Part print with two shaded views. Sizes in mm from the minimum x, y, z corner. A direction names the side the tool comes from. Round coordinates to 2 decimals unless told otherwise and drop trailing zeros. Write each loop counter-clockwise with the first axis right and the second up, starting at its lowest first coordinate (ties: lowest second). Pieces come first, ordered by that corner, then holes. Notation, with made-up numbers: (-32, 1) -> (-15, 1) arc R31 ccw to (-15, 37) -> close; hole circle Ø2 at (-33.5, -35.5). An arc over 180 degrees is marked (long way). Answer in a Markdown table with one row per item. Add a question column.
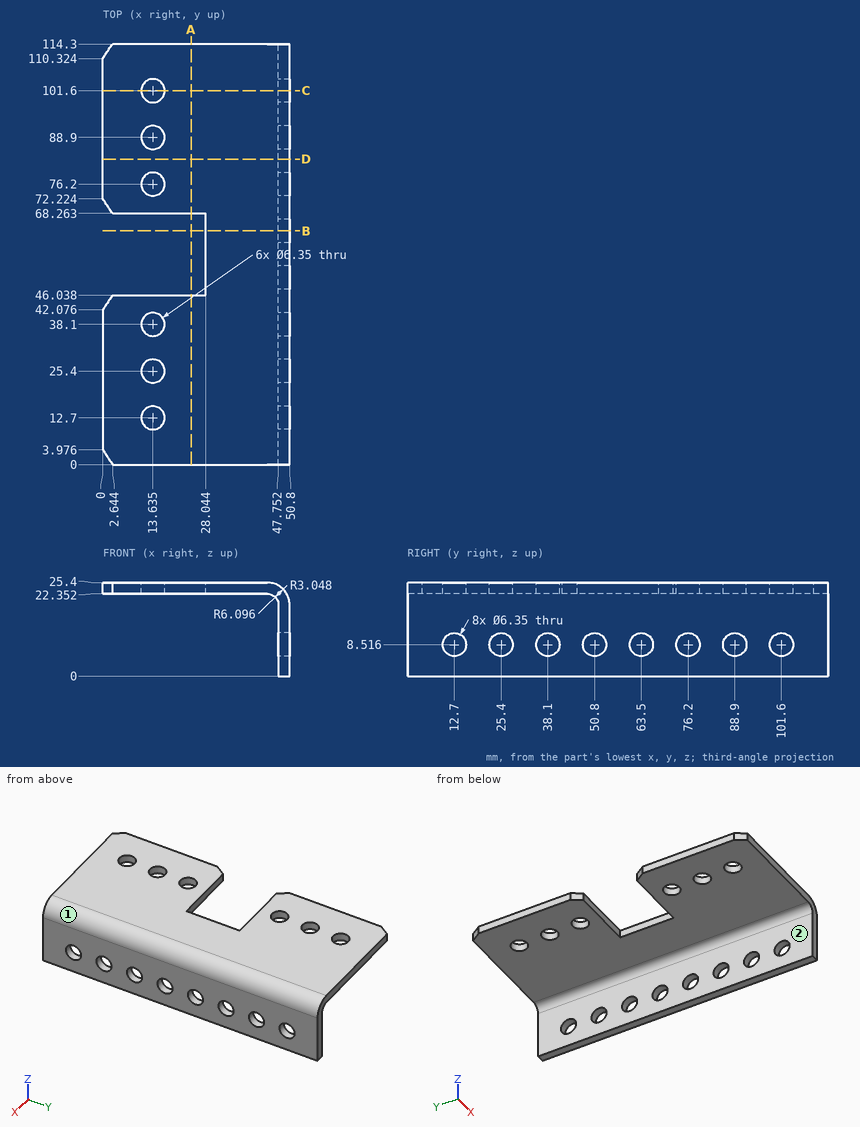
Item 1: Tool access for the marked faces 1 and 2: list every direction of +Z, -Z, +X, -X, +Y, -Y with a clear straight run to the whole face (end or side of a thin tool).
Item 2: Saw through at D-D on y = 83. Give the cut face in (x, z) (1 decimal), then the cut area to 3 significant figures.
Item 3: Saw through at B-B on y = 63.5. Give the cut face in (x, z) (1 decimal).
Item 4: Drill centre lines: probe 1 along X at (y, z) = (35, 7.25); probe 2 along Z at (x, y) = (20, 69); probe 3 along X at (y, z) = (106, 19.5) (1 decimal). Where is each one in solid material? Low to high.
Item 5: Pin check, flat tips, straight feed: pin 1 (8.5 mm diameter, centred on y = 76.2, z = 8.52, fed in from -X); pin 2 (10 mm diameter, centred on x = 7, y = 92.5, fed in from -Z); pin 3 (2.5 mm diameter, centred on y = 56.5, z = 23.5, fed in from -X). Stop position of each tip, or through.
Item 6: Saw through at A-A on x = 24. Give the cut face in (y, z).
Item 7: Saw through at C-C on y = 101.6. Give the cut face in (x, z) (1 decimal), then the cut area to 3 significant figures.
Recorded:
| question | item | result |
|---|---|---|
| 1 | face 1 | +Z, +X, +Y, -Y |
| 1 | face 2 | -Z, -X, +Y, -Y |
| 2 | outline | (0, 22.4) -> (44.7, 22.4) arc R3 cw to (47.8, 19.3) -> (47.8, 0) -> (50.8, 0) -> (50.8, 19.3) arc R6.1 ccw to (44.7, 25.4) -> (0, 25.4) -> close |
| 2 | area | 217 mm2 |
| 3 | outline | (28, 22.4) -> (44.7, 22.4) arc R3 cw to (47.8, 19.3) -> (47.8, 11.7) -> (50.8, 11.7) -> (50.8, 19.3) arc R6.1 ccw to (44.7, 25.4) -> (28, 25.4) -> close; (47.8, 0) -> (50.8, 0) -> (50.8, 5.3) -> (47.8, 5.3) -> close |
| 4 | probe 1 | 47.75 to 50.8 |
| 4 | probe 2 | 22.35 to 25.4 |
| 4 | probe 3 | 47.7 to 50.8 |
| 5 | pin 1 | x = 47.75 |
| 5 | pin 2 | z = 22.35 |
| 5 | pin 3 | x = 28.04 |
| 6 | outline | (0, 22.35) -> (46.04, 22.35) -> (46.04, 25.4) -> (0, 25.4) -> close; (68.26, 22.35) -> (114.3, 22.35) -> (114.3, 25.4) -> (68.26, 25.4) -> close |
| 7 | outline | (0, 22.4) -> (10.5, 22.4) -> (10.5, 25.4) -> (0, 25.4) -> close; (16.8, 22.4) -> (44.7, 22.4) arc R3 cw to (47.8, 19.3) -> (47.8, 11.7) -> (50.8, 11.7) -> (50.8, 19.3) arc R6.1 ccw to (44.7, 25.4) -> (16.8, 25.4) -> close; (47.8, 0) -> (50.8, 0) -> (50.8, 5.3) -> (47.8, 5.3) -> close |
| 7 | area | 178 mm2 |
